The listing builds one solid part. Answer for the finished solid, in the listing's coordinates (mm). Face numbers are marked on the shaded views. Give positions to 0.01 mm unless a question says otherwise; leave off trailing zeros. Write each loop counter-clockwise with the first axis right and the second up, starting at its lowest first coordinate (ties: lowest second). Pieces come first, ordered by that corner, then holes. Notation, with made-up numbers: (53.5, -15.75) - (96.5, -15.75) arc R20 cw to (96.5, 23.25) - close; hole circle Ø8 at (9.5, -11). An arc over 180 degrees is marked (long way). Write each question's results on one line, items separated by ' | '. Start each with the question number.
Q1. Section C-C (y = 10.25) is taken. Determine the outline of the cut face in (x, z), plus the area to 3 significant figures.
Q2. Section A-A (z = 0) is taken. Determine the outline of the cut face in (x, y), plus the area to 3 significant figures.
Q3. Find the intervals of material crossed by probe 1 along X at (y, z) = (1.95, 0); probe 2 along Y at (x, z) = (5, 8.5); probe 3 along X at (y, z) = (10.25, 0), in increasing order.
Q4. For a pull along X with two mould halves and no side action, classify the marked faces 1, 2 and 3 as pulls with the +X half, pulls with the -X half, needs draft (parallel to the pull), parting line crosses it, or undercut.
Q5. Section B-B (x = 0) is taken. Determine the outline of the cut face in (y, z), plus the area to 3 significant figures.
Q6. Flat-ended cylindrical pins translate along their axes: pin 1 Ø4.5 at (x, z) = (0, 12) entering from +Y; pin 2 Ø4 at (x, y) = (3.5, 2.5) entering from -Z; pin 3 Ø5 at (x, y) = (-12, 2.5) entering from +Z. Find the tip coordinate at first contact, or state that the pin passes through.
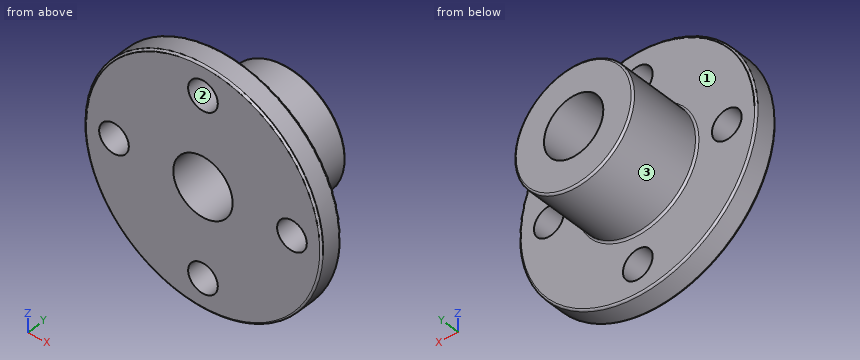
```python
from build123d import *

# Parameters (mm, degrees)
SKETCH1_R           = 16
BOSS_EXTRUDE1_DEPTH = 3
FILLET1_R           = 0.25
SKETCH2_R           = 8
BOSS_EXTRUDE2_DEPTH = 10
FILLET2_R           = 0.25
CUT_EXTRUDE1_REACH  = 28.096
SKETCH3_R           = 4
CUT_EXTRUDE2_REACH  = 26.739
SKETCH4_R           = 2


with BuildPart() as part:
    # Sketch1 → Boss-Extrude1 (new body)
    with BuildSketch(Plane(origin=(0, 0, 0), x_dir=(1, 0, 0), z_dir=(0, 1, 0))):
        with Locations(Location((0, 0, 0), (0, 0, 270))):
            Circle(SKETCH1_R)
    extrude(amount=BOSS_EXTRUDE1_DEPTH)

    # Fillet1
    fillet1_edges = [part.edges().sort_by_distance(p)[0] for p in [
        (0, 0, -16),
        (0, 3, -16),
    ]]
    fillet(fillet1_edges, radius=FILLET1_R)

    # Sketch2 → Boss-Extrude2 (add)
    with BuildSketch(Plane(origin=(0, 3, 0), x_dir=(1, 0, 0), z_dir=(0, 1, 0))):
        with Locations(Location((0, 0, 0), (0, 0, 270))):
            Circle(SKETCH2_R)
    extrude(amount=BOSS_EXTRUDE2_DEPTH)

    # Fillet2
    fillet2_edges = [part.edges().sort_by_distance(p)[0] for p in [
        (0, 3, -8),
        (0, 13, -8),
    ]]
    fillet(fillet2_edges, radius=FILLET2_R)

    # Sketch3 → Cut-Extrude1 (cut, up to next)
    with BuildSketch(Plane(origin=(0, 13, 0), x_dir=(1, 0, 0), z_dir=(0, 1, 0)), mode=Mode.PRIVATE) as cut_extrude1_sk1:
        with Locations(Location((0, 0, 0), (0, 0, 270))):
            Circle(SKETCH3_R)
    cut_extrude1_tool1 = extrude(cut_extrude1_sk1.sketch, amount=-CUT_EXTRUDE1_REACH, mode=Mode.PRIVATE) & part.part
    add(cut_extrude1_tool1.solids().sort_by_distance((0, 13, 0))[0], mode=Mode.SUBTRACT)

    # Sketch4 → Cut-Extrude2 (cut, up to next)
    with BuildSketch(Plane(origin=(0, 3, 0), x_dir=(1, 0, 0), z_dir=(0, 1, 0)), mode=Mode.PRIVATE) as cut_extrude2_sk1:
        with Locations(Location((0, 12, 0), (0, 0, 270))):
            Circle(SKETCH4_R)
    cut_extrude2_tool1 = extrude(cut_extrude2_sk1.sketch, amount=-CUT_EXTRUDE2_REACH, mode=Mode.PRIVATE) & part.part
    # Sketch4 → Cut-Extrude2 (cut, up to next)
    with BuildSketch(Plane(origin=(0, 3, 0), x_dir=(1, 0, 0), z_dir=(0, 1, 0)), mode=Mode.PRIVATE) as cut_extrude2_sk2:
        with Locations(Location((-12, 0, 0), (0, 0, 270))):
            Circle(SKETCH4_R)
    cut_extrude2_tool2 = extrude(cut_extrude2_sk2.sketch, amount=-CUT_EXTRUDE2_REACH, mode=Mode.PRIVATE) & part.part
    # Sketch4 → Cut-Extrude2 (cut, up to next)
    with BuildSketch(Plane(origin=(0, 3, 0), x_dir=(1, 0, 0), z_dir=(0, 1, 0)), mode=Mode.PRIVATE) as cut_extrude2_sk3:
        with Locations(Location((0, -12, 0), (0, 0, 270))):
            Circle(SKETCH4_R)
    cut_extrude2_tool3 = extrude(cut_extrude2_sk3.sketch, amount=-CUT_EXTRUDE2_REACH, mode=Mode.PRIVATE) & part.part
    # Sketch4 → Cut-Extrude2 (cut, up to next)
    with BuildSketch(Plane(origin=(0, 3, 0), x_dir=(1, 0, 0), z_dir=(0, 1, 0)), mode=Mode.PRIVATE) as cut_extrude2_sk4:
        with Locations(Location((12, 0, 0), (0, 0, 270))):
            Circle(SKETCH4_R)
    cut_extrude2_tool4 = extrude(cut_extrude2_sk4.sketch, amount=-CUT_EXTRUDE2_REACH, mode=Mode.PRIVATE) & part.part
    add(cut_extrude2_tool1.solids().sort_by_distance((0, 3, -12))[0], mode=Mode.SUBTRACT)
    add(cut_extrude2_tool2.solids().sort_by_distance((-12, 3, 0))[0], mode=Mode.SUBTRACT)
    add(cut_extrude2_tool3.solids().sort_by_distance((0, 3, 12))[0], mode=Mode.SUBTRACT)
    add(cut_extrude2_tool4.solids().sort_by_distance((12, 3, 0))[0], mode=Mode.SUBTRACT)


solid = part.part
```
Answers below:
1) outline: circle Ø16 at (0, 0); hole circle Ø8 at (0, 0) | area: 151 mm2
2) outline: (-16, 0.25) arc R0.25 ccw to (-15.75, 0) - (-14, 0) - (-14, 3) - (-15.75, 3) arc R0.25 ccw to (-16, 2.75) - close; (-10, 0) - (-4, 0) - (-4, 13) - (-7.75, 13) arc R0.25 ccw to (-8, 12.75) - (-8, 3.25) arc R0.25 cw to (-8.25, 3) - (-10, 3) - close; (4, 0) - (10, 0) - (10, 3) - (8.25, 3) arc R0.25 cw to (8, 3.25) - (8, 12.75) arc R0.25 ccw to (7.75, 13) - (4, 13) - close; (14, 0) - (15.75, 0) arc R0.25 ccw to (16, 0.25) - (16, 2.75) arc R0.25 ccw to (15.75, 3) - (14, 3) - close | area: 128 mm2
3) probe 1: x = -16 to -14, -10 to -4, 4 to 10, 14 to 16 | probe 2: y = 0 to 3 | probe 3: x = -8 to -4, 4 to 8
4) face 1: needs draft | face 2: undercut | face 3: parting line crosses it
5) outline: (0, -15.75) arc R0.25 ccw to (0.25, -16) - (2.75, -16) arc R0.25 ccw to (3, -15.75) - (3, -14) - (0, -14) - close; (0, -10) - (3, -10) - (3, -8.25) arc R0.25 cw to (3.25, -8) - (12.75, -8) arc R0.25 ccw to (13, -7.75) - (13, -4) - (0, -4) - close; (0, 4) - (13, 4) - (13, 7.75) arc R0.25 ccw to (12.75, 8) - (3.25, 8) arc R0.25 cw to (3, 8.25) - (3, 10) - (0, 10) - close; (0, 14) - (3, 14) - (3, 15.75) arc R0.25 ccw to (2.75, 16) - (0.25, 16) arc R0.25 ccw to (0, 15.75) - close | area: 128 mm2
6) pin 1: stops at y = 3 | pin 2: stops at z = -15.93 | pin 3: stops at z = 12.87
